```python
from build123d import *

# Parameters (mm, degrees)
SKETCH1_R           = 2
BOSS_EXTRUDE1_DEPTH = 1.5
SKETCH2_W           = 45
SKETCH2_H           = 1.5
BOSS_EXTRUDE2_DEPTH = 4.5
FILLET1_R           = 3


with BuildPart() as part:
    # Sketch1 → Boss-Extrude1 (new body)
    with BuildSketch(Plane(origin=(0, 0, 0), x_dir=(1, 0, 0), z_dir=(0, 1, 0))):
        with BuildLine():
            Line((-22.5, 9), (22.5, 9))
            Line((22.5, 9), (22.5, 1))
            ThreePointArc((22.5, 1), (21.035533906, -2.535533906), (17.5, -4))
            Line((17.5, -4), (-17.5, -4))
            ThreePointArc((-17.5, -4), (-21.035533906, -2.535533906), (-22.5, 1))
            Line((-22.5, 1), (-22.5, 9))
        make_face()
        with Locations(Location((0, 0, 0), (0, 0, 270))):
            Circle(SKETCH1_R, mode=Mode.SUBTRACT)
    extrude(amount=BOSS_EXTRUDE1_DEPTH)

    # Sketch2 → Boss-Extrude2 (add)
    with BuildSketch(Plane(origin=(0, 1.5, 0), x_dir=(1, 0, 0), z_dir=(0, 1, 0))):
        with Locations((0, 8.25)):
            Rectangle(SKETCH2_W, SKETCH2_H)
    extrude(amount=BOSS_EXTRUDE2_DEPTH)

    # Fillet1
    fillet1_edges = [part.edges().sort_by_distance(p)[0] for p in [
        (0, 1.5, -7.5),
    ]]
    fillet(fillet1_edges, radius=FILLET1_R)


solid = part.part
```
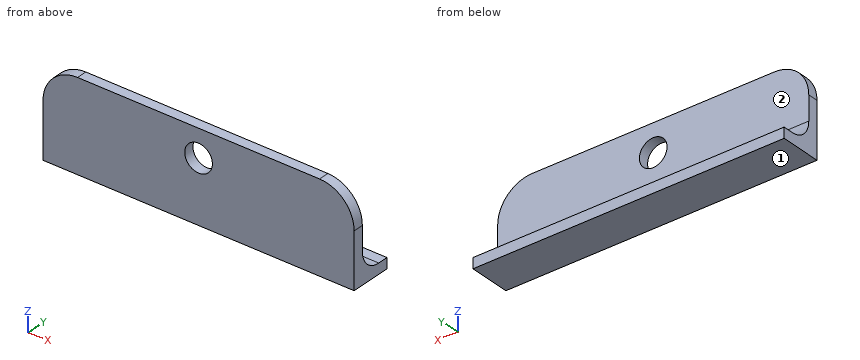
For this review, take the finished solid that the model builds, in its own axes (mm). Face numbers are marked on the shaded views. A direction names the side the tool comes from. Give positions to 0.01 mm unless a question says otherwise; leave off trailing zeros. Write each loop counter-clockwise with the first axis right and the second up, starting at its lowest first coordinate (ties: lowest second). Pieces come first, ordered by that corner, then holes.
Item 1: Take a section at B-B (x = 0). Give the boundary of the cut face in (y, z), and give its area (3 significant figures).
Item 2: Wall thickness on probe 1 along Z at (x, y) = (-20, 4.65); probe 2 along Y at (x, z) = (19.5, 1.5); probe 3 along X at (y, z) = (0.85, 0): over which ranges is each line inside the solid? List them lowest first.
Item 3: Take a section at C-C (y = 5.35). Give the boundary of the cut face in (x, z).
Item 4: Machinability: for the marked faces 1 and 2, which of the approach directions +Z, -Z, +X, -X, +Y, -Y give a long, thin tool a straight path to every point of the face, cutting with its end or side? Answer none if there is none.
Item 5: Take a section at A-A (z = 0). Give the boundary of the cut face in (x, y), and give its area (3 significant figures).
Item 6: Take a section at D-D (x = -12). Give the boundary of the cut face in (y, z), and give its area (3 significant figures).
Item 7: Insertion check: P1, Ø3, axis at x = -16, z = -5.5, coming from the +Y side; P2, Ø1.5, axis at x = -3.5, z = -4, coming from the -Y side; P3, Ø3.5, axis at x = 0, z = 0, coming from the +Y side; P4, Ø1.2, axis at x = -5, y = 5.5, coming from the +Z side. Each pin has a flat end and moves straight along its axis. Give the tip position at first contact, or say it passes through.
Established:
1. outline: (0, -9) - (6, -9) - (6, -7.5) - (4.5, -7.5) arc R3 cw to (1.5, -4.5) - (1.5, -2) - (0, -2) - close; (0, 2) - (1.5, 2) - (1.5, 4) - (0, 4) - close
1. area: 22.2 mm2
2. probe 1: z = -9 to -7.5
2. probe 2: y = 0 to 1.5
2. probe 3: x = -22.4 to -2, 2 to 22.4
3. outline: (-22.5, -9) - (22.5, -9) - (22.5, -7.5) - (-22.5, -7.5) - close
4. face 1: -Z, +X, -X, +Y, -Y
4. face 2: +Z, +X, -X, +Y
5. outline: (-22.4, 0) - (-2, 0) - (-2, 1.5) - (-22.4, 1.5) - close; (2, 0) - (22.4, 0) - (22.4, 1.5) - (2, 1.5) - close
5. area: 61.2 mm2
6. outline: (0, -9) - (6, -9) - (6, -7.5) - (4.5, -7.5) arc R3 cw to (1.5, -4.5) - (1.5, 4) - (0, 4) - close
6. area: 28.2 mm2
7. P1: stops at y = 2.84
7. P2: stops at y = 0
7. P3: passes through
7. P4: stops at z = -7.5
